The drawing under review shows one solid part. Ordinate dimensions are in mm from its lowest x, y, z. Round coordinates to 2 decimals unless told otherwise and drop trailing zeros. Order: outer loops, then holes, each group sorted by start corner. A loop starts at its lowest first (then second) coordinate and runs counter-clockwise, first axis right, second up. Notation, with made-up numbers: M 11.25,18 L 58.25,18 A25 cw 58.25,39 Z; hole C -26.5,62.5 d8. An arc over 180 degrees is marked long. Answer as a JSON object with one key per item and string values.
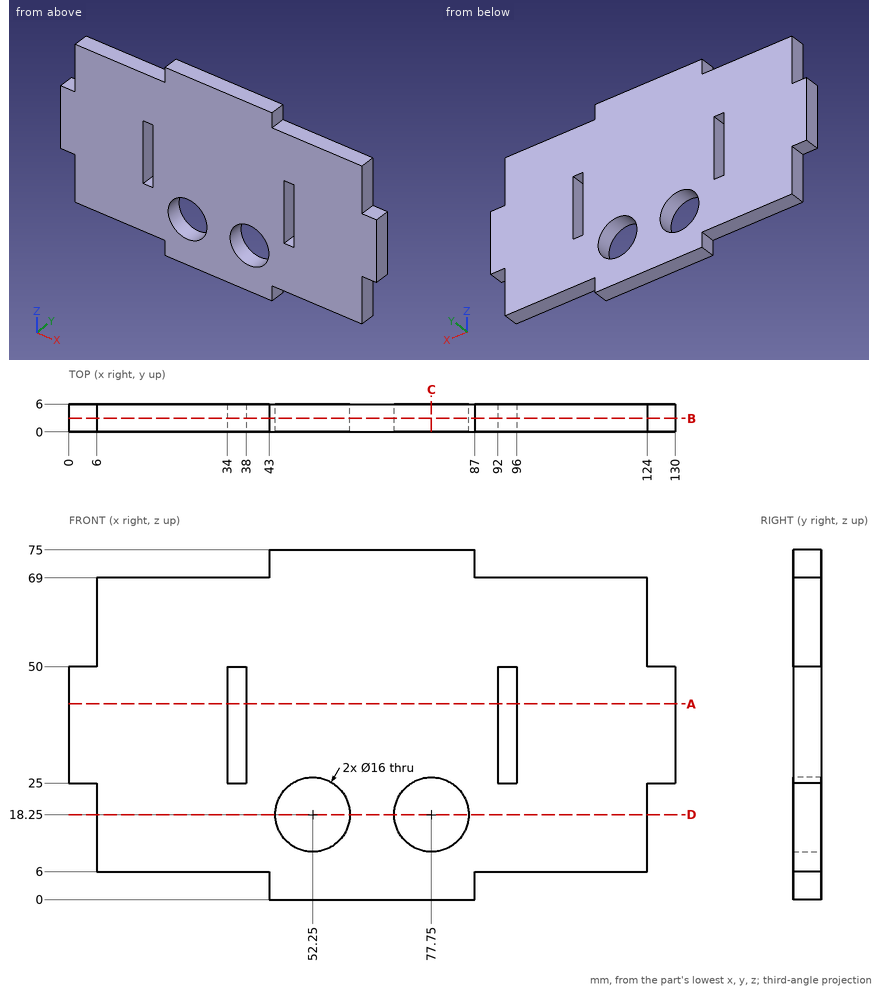
1) For L1, parallel to X at y = 4, z = 18.25; L2, parallel to X at y = 4.5, z = 33; L3, parallel to Z at x = 125, y = 4.95, list the stretches that pass through material, from the lowest coordinate up.
Geometry check:
{"L1": "x = 6 to 44.25, 60.25 to 69.75, 85.75 to 124", "L2": "x = 0 to 34, 38 to 92, 96 to 130", "L3": "z = 25 to 50"}
2) Add section A-A on z = 42. State the section outline as (x, y) points.
Geometry check:
{"outline": "M 0,0 L 34,0 L 34,6 L 0,6 Z; M 38,0 L 92,0 L 92,6 L 38,6 Z; M 96,0 L 130,0 L 130,6 L 96,6 Z"}
3) Add section C-C on x = 77.75. State the section outline as (y, z) points.
Geometry check:
{"outline": "M 0,0 L 6,0 L 6,10.25 L 0,10.25 Z; M 0,26.25 L 6,26.25 L 6,75 L 0,75 Z"}
4) Add section D-D on z = 18.25. State the section outline as (x, y) points, and give its area (3 significant figures).
Geometry check:
{"outline": "M 6,0 L 44.25,0 L 44.25,6 L 6,6 Z; M 60.25,0 L 69.75,0 L 69.75,6 L 60.25,6 Z; M 85.75,0 L 124,0 L 124,6 L 85.75,6 Z", "area": "516 mm²"}
5) Insertion check: P1, Ø3, axis at x = 127, y = 4, coming from the +Z side; P2, Ø1.2, axis at x = 94.5, y = 3.5, coming from the +Z side; P3, Ø3, axis at x = 109, y = 2, coming from the -Z side. Each pin has a flat end and moves straight along its axis. Give the tip position at first contact, or say it passes through.
Geometry check:
{"P1": "stops at z = 50", "P2": "stops at z = 69", "P3": "stops at z = 6"}
6) Add section B-B on y = 2.9. State how many separate pieces and enclosed holes the cut face has, and give its area (3 significant figures).
Geometry check:
{"separate pieces": "1", "enclosed holes": "4", "area": "7,660 mm²"}
